from build123d import *

# Parameters (mm, degrees)
SKETCH1_R           = 2.5
BOSS_EXTRUDE1_DEPTH = 6.2


with BuildPart() as part:
    # Sketch1 → Boss-Extrude1 (new body)
    with BuildSketch(Plane.XY):
        with BuildLine():
            Line((-116.938372425, -13.911569107), (-87, -22.25))
            ThreePointArc((-87, -22.25), (-77.031989093, -24.309319739), (-66.876941087, -25))
            Line((-66.876941087, -25), (65, -25))
            ThreePointArc((65, -25), (75.977025607, -24.261995409), (86.756474933, -22.061265033))
            Line((86.756474933, -22.061265033), (114.235144317, -14.5))
            ThreePointArc((114.235144317, -14.5), (120.463338609, -13.323456153), (126.8, -13.177230394))
            ThreePointArc((126.8, -13.177230394), (140.274563377, 3.600104754), (120, 10.810161116))
            ThreePointArc((120, 10.810161116), (96.313236011, -2.023267975), (70.328890052, -9.134769615))
            ThreePointArc((70.328890052, -9.134769615), (64.680941239, -9.783377892), (59, -10))
            Line((59, -10), (-59, -10))
            ThreePointArc((-59, -10), (-66.518658645, -9.998172905), (-74, -9.25))
            ThreePointArc((-74, -9.25), (-98.410939741, -2.539404949), (-120.554503776, 9.732051233))
            ThreePointArc((-120.554503776, 9.732051233), (-138.868880222, 4.055609252), (-128.349445963, -11.974982784))
            ThreePointArc((-128.349445963, -11.974982784), (-122.593742509, -12.647675527), (-116.938372425, -13.911569107))
        make_face()
        with Locations(Location((127.574986581, 0, 0), (0, 0, 180))):
            Circle(SKETCH1_R, mode=Mode.SUBTRACT)
        with Locations(Location((-127.574986581, 0, 0), (0, 0, 180))):
            Circle(SKETCH1_R, mode=Mode.SUBTRACT)
    extrude(amount=BOSS_EXTRUDE1_DEPTH)


solid = part.part
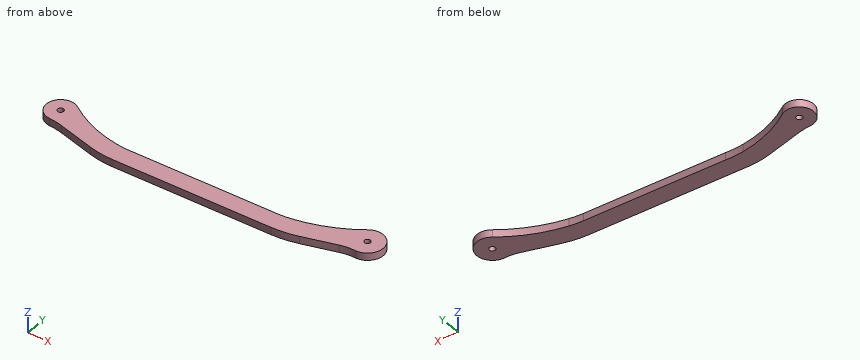
The listing builds one solid part. Answer for the finished solid, in the listing's coordinates (mm). Coordinates: 2 decimals unless noted, no trailing zeros. Loops run counter-clockwise (first coordinate to the right, second up) from the corner with the lowest first, then second, coordinate; pieces in that order, holes last.
1) Find the intervals of material crossed by L1, parallel to X at y = -1, z = 3; L2, parallel to Y at x = -53.5, z = 3.75; L3, parallel to X at y = 6.5, z = 3, in increasing order.
2) Flat-ended cylindrical pins translate along their axes: pin 1 Ø3 at (x, z) = (-77.5, 2) entering from -Y; pin 2 Ø2 at (y, z) = (-8.5, 1) entering from -X; pin 3 Ø3 at (x, z) = (11, 3.5) entering from +Y. Find the tip coordinate at first contact, or state that the pin passes through.
3) Find section D-D on y = -17.5. Write down the section's boundary in (x, z).
4) Find section A-A on y = 0. Write down the section's boundary in (x, z), then the cut area to 3 significant figures.
5) Find section B-B on x = -43. Write down the section's boundary in (y, z), then the cut area to 3 significant figures.
6) Find section C-C on z = 3.25. Write down the section's boundary in (x, y), then the cut area to 3 significant figures.
Values:
1. L1: x = -139.53 to -129.87, -125.28 to -102, 98.78 to 125.28, 129.87 to 140.74
1. L2: y = -25 to -10
1. L3: x = -137.66 to -115.81, 113.39 to 139.06
2. pin 1: stops at y = -24.44
2. pin 2: stops at x = -136.94
2. pin 3: stops at y = -10
3. outline: (-104.05, 0) - (103.33, 0) - (103.33, 6.2) - (-104.05, 6.2) - close
4. outline: (-139.57, 0) - (-130.07, 0) - (-130.07, 6.2) - (-139.57, 6.2) - close; (-125.07, 0) - (-104.15, 0) - (-104.15, 6.2) - (-125.07, 6.2) - close; (101.05, 0) - (125.07, 0) - (125.07, 6.2) - (101.05, 6.2) - close; (130.07, 0) - (140.77, 0) - (140.77, 6.2) - (130.07, 6.2) - close
4. area: 404 mm2
5. outline: (-25, 0) - (-10, 0) - (-10, 6.2) - (-25, 6.2) - close
5. area: 93.0 mm2
6. outline: (-128.35, -11.97) arc R56 cw to (-116.94, -13.91) - (-87, -22.25) arc R75 ccw to (-66.88, -25) - (65, -25) arc R82 ccw to (86.76, -22.06) - (114.24, -14.5) arc R38.78 cw to (126.8, -13.18) arc R13.2 ccw (long way) to (120, 10.81) arc R117.7 cw to (70.33, -9.13) arc R74.6 cw to (59, -10) - (-59, -10) arc R75.65 cw to (-74, -9.25) arc R106.73 cw to (-120.55, 9.73) arc R12 ccw (long way) to start; hole circle Ø5 at (-127.57, 0); hole circle Ø5 at (127.57, 0)
6. area: 4,700 mm2
